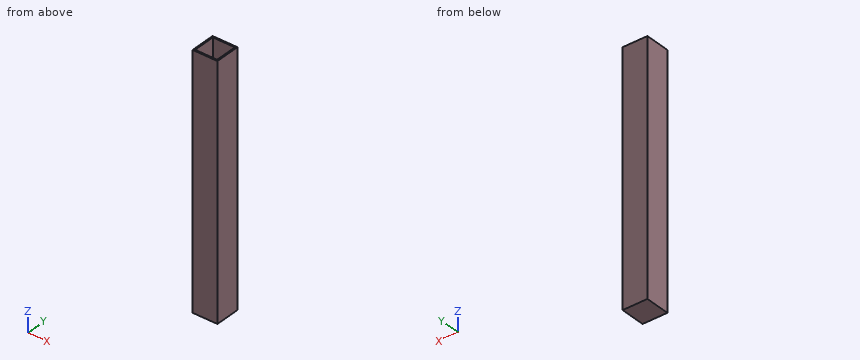
Autodesk Inventor part; units mm, degrees
ref_plane "YZ Plane" through (0, 0, 0) normal (1, 0, 0) x (0, 1, 0)
ref_plane "XZ Plane" through (0, 0, 0) normal (0, 1, 0) x (-1, 0, 0)
ref_plane "XY Plane" through (0, 0, 0) normal (0, 0, 1) x (1, 0, 0)
sketch "Sketch1" plane through (0, 0, 0) normal (0, 0, 1) x (1, 0, 0)
  line L0 (-31.9903, -7.2804) -> (-1.9903, -7.2804)
  line L1 (-1.9903, -7.2804) -> (-1.9903, 22.7196)
  line L2 (-1.9903, 22.7196) -> (-31.9903, 22.7196)
  line L3 (-31.9903, -7.2804) -> (-31.9903, 22.7196)
  line L4 (-30.2903, 22.7196) -> (-30.2903, -7.2804)
  line L5 (-31.9903, -5.5804) -> (-1.9903, -5.5804)
  line L6 (-3.6903, 22.7196) -> (-3.6903, -7.2804)
  line L7 (-31.9903, 21.0196) -> (-1.9903, 21.0196)
  point P0 (0, 0)
  point P1 (-3.6903, 21.0196)
  point P2 (-30.2903, 21.0196)
  point P3 (-30.2903, -5.5804)
  point P4 (-3.6903, -5.5804)
  dimension "d0" = 30
  dimension "d1" = 30
  dimension "d2" = 1.7
  dimension "d3" = 1.7
  dimension "d4" = 1.7
  dimension "d5" = 1.7
extrude "Extrusion1" add sketch "Sketch1" against normal blind 298.722
extrude "Extrusion2" cut sketch "Sketch1" against normal blind 278.523 contours L4 L7 L6 L5
properties part number "Cablecanal Ranurado 30x30 L=115 mm" material "PVC-Piping"
Check sheet for the modelled part. Datum: model origin and axes. Units: mm. Coordinates: 2 decimals unless noted, no trailing zeros. Write each loop counter-clockwise with the first axis right and the second up, starting at its lowest first coordinate (ties: lowest second). Pieces come first, ordered by that corner, then holes. Notation, with made-up numbers: (88.25, -10) -> (131.25, -10) arc R20 cw to (131.25, 17) -> close; hole circle Ø10 at (-17, 5.25). An arc over 180 degrees is marked (long way). Use a Markdown table: item, result.
1. Scan lines: line 1 along X through (y, z) = (15.5, -206); line 2 along Y through (x, z) = (-29, -69); line 3 along Z through (x, y) = (-7.75, 6). Record each from-to range of solid material in increasing order.
Reported:
| item | result |
|---|---|
| line 1 | x = -31.99 to -30.29, -3.69 to -1.99 |
| line 2 | y = -7.28 to -5.58, 21.02 to 22.72 |
| line 3 | z = -298.72 to -278.52 |
2. Sectioned sample at A-A (x = -23.75). Enter the section's corners in (y, z).
Reported:
| item | result |
|---|---|
| outline | (-7.28, -298.72) -> (22.72, -298.72) -> (22.72, 0) -> (21.02, 0) -> (21.02, -278.52) -> (-5.58, -278.52) -> (-5.58, 0) -> (-7.28, 0) -> close |
3. Sectioned sample at B-B (z = -265). Enter the section's corners in (x, y), plus the area to 3 significant figures.
Reported:
| item | result |
|---|---|
| outline | (-31.99, -7.28) -> (-1.99, -7.28) -> (-1.99, 22.72) -> (-31.99, 22.72) -> close; hole (-30.29, -5.58) -> (-3.69, -5.58) -> (-3.69, 21.02) -> (-30.29, 21.02) -> close |
| area | 192 mm2 |
4. Go/stop test with a flat-tipped pin: pin 1 Ø1.5 at (x, y) = (-28.5, 18) entering from +Z. Record where the tip stops, or that it passes through.
Reported:
| item | result |
|---|---|
| pin 1 | stops at z = -278.52 |
5. Sectioned sample at C-C (y = 7.25). Enter the section's corners in (x, z), plus the area to 3 significant figures.
Reported:
| item | result |
|---|---|
| outline | (-31.99, -298.72) -> (-1.99, -298.72) -> (-1.99, 0) -> (-3.69, 0) -> (-3.69, -278.52) -> (-30.29, -278.52) -> (-30.29, 0) -> (-31.99, 0) -> close |
| area | 1,550 mm2 |
